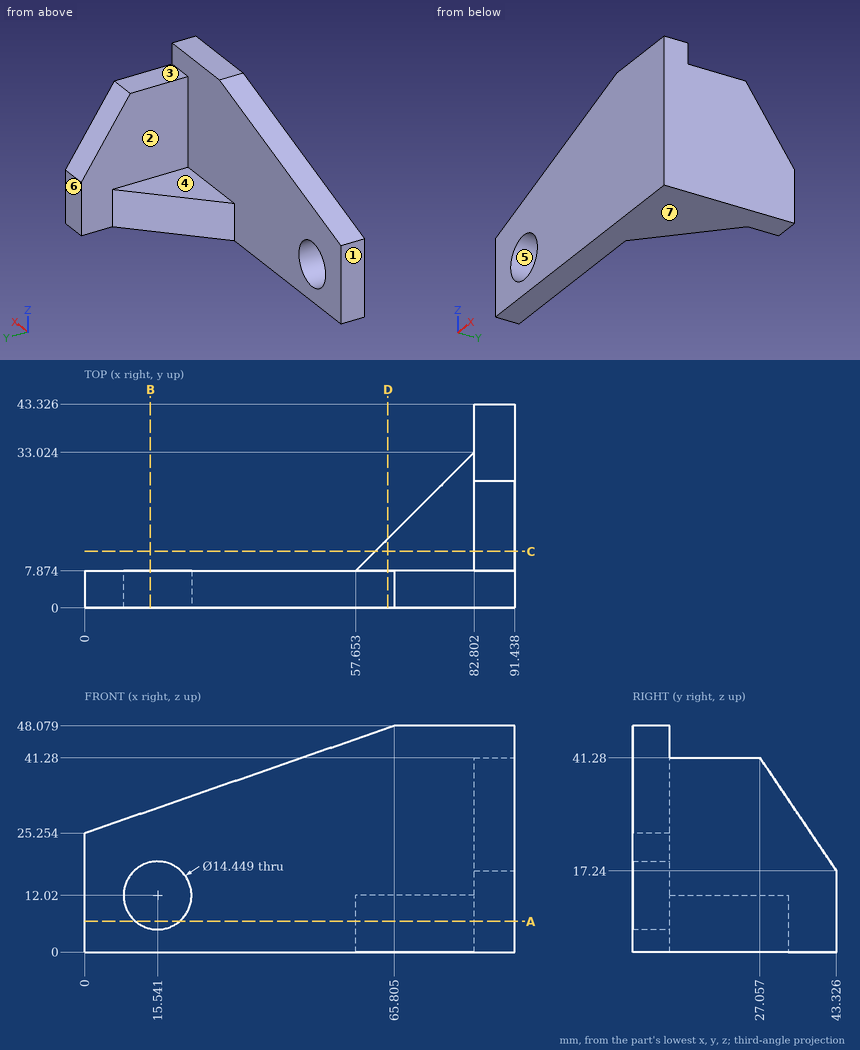
Could you check a few things on this drawing? It's one solid part, dimensions in mm from its lowest x, y, z. A direction names the side the tool comes from. Coordinates: 2 decimals unless noted, no trailing zeros. Write each loop counter-clockwise with the first axis right and the second up, starting at its lowest first coordinate (ties: lowest second). Pieces come first, ordered by that corner, then holes.
Q1. Imagine slicing it at B-B, the plane x = 14. List the corners of the cut face in (y, z) for me.
Results found:
outline: (0, 0) - (7.87, 0) - (7.87, 4.96) - (0, 4.96) - close; (0, 19.08) - (7.87, 19.08) - (7.87, 30.11) - (0, 30.11) - close
Q2. Imagine slicing it at A-A, the plane z = 6.5. List the corners of the cut face in (x, y) for me.
Results found:
outline: (0, 0) - (10.88, 0) - (10.88, 7.87) - (0, 7.87) - close; (20.2, 0) - (91.44, 0) - (91.44, 43.33) - (82.8, 43.33) - (82.8, 33.02) - (57.65, 7.87) - (20.2, 7.87) - close
Q3. If we mould it in two halves opening along Z, with no side actions, what happens to the marked faces 4, 5, 6 and 7? For each: +Z half, -Z half, draft (parallel to the pull), parting line (faces both ways), or undercut.
Results found:
face 4: +Z half
face 5: undercut
face 6: draft
face 7: -Z half
Q4. Imagine slicing it at D-D, the plane x = 64.5. List the corners of the cut face in (y, z) for me, plus the area to 3 significant figures.
Results found:
outline: (0, 0) - (14.72, 0) - (14.72, 12.02) - (7.87, 12.02) - (7.87, 47.63) - (0, 47.63) - close
area: 457 mm2
Q5. Imagine slicing it at C-C, the plane y = 12. List the corners of the cut face in (x, z) for me, plus the area to 3 significant figures.
Results found:
outline: (61.78, 0) - (91.44, 0) - (91.44, 41.28) - (82.8, 41.28) - (82.8, 12.02) - (61.78, 12.02) - close
area: 609 mm2
Q6. For P1, Ø1.5, axis at y = 22, z = 16, coming from the -X side; P2, Ø7.5, axis at x = 67, y = 17, coming from the +Z side; P3, Ø4, axis at x = 61.5, z = 8.5, coming from the +Y side, each with a flat end and sliding along its axis, tell me the tip position at first contact or that it passes through.
Results found:
P1: stops at x = 82.8
P2: stops at z = 12.02
P3: stops at y = 13.72
Q7. Please list where these lines run through material, in increasing order: L1, parallel to X at y = 14, z = 30; L2, parallel to Y at x = 35.5, z = 20; L3, parallel to Z at x = 75, y = 20.5.
Results found:
L1: x = 82.8 to 91.44
L2: y = 0 to 7.87
L3: z = 0 to 12.02
Q8. Which directions (+Z, -Z, +X, -X, +Y, -Y) give clear straight access to the entire face, cutting with the end or side of a thin tool? Please do the marked faces 1, 2 and 3.
Results found:
face 1: +Z, -Z, -X, +Y, -Y
face 2: +Z, -X, +Y
face 3: +Z, +X, -X, +Y
